from build123d import *

# Parameters (mm, degrees)
SKETCH1_W               = 160
SKETCH1_H               = 129
BOSS_EXTRUDE1_DEPTH     = 8
SKETCH1_3_R             = 4
CUT_EXTRUDE2_DEPTH      = 104.074002542
FILLET1_R               = 10
CUT_EXTRUDE4_DEPTH      = 1
CUT_EXTRUDE4_DEPTH_BACK = 3
CUT_EXTRUDE4_START      = 8
CUT_EXTRUDE9_DEPTH      = 104.074002542
CUT_EXTRUDE10_START     = 8
SKETCH1_17_R            = 2.5
SKETCH1_17_R_2          = 10
CUT_EXTRUDE10_DEPTH     = 5
BOSS_EXTRUDE4_START     = 10
BOSS_EXTRUDE4_DEPTH     = 10
FILLET2_R               = 10


with BuildPart() as part:
    # Sketch1 → Boss-Extrude1 (new body)
    with BuildSketch(Plane(origin=(0, 0, 0), x_dir=(1, 0, 0), z_dir=(0, 1, 0))):
        Rectangle(SKETCH1_W, SKETCH1_H)
    extrude(amount=BOSS_EXTRUDE1_DEPTH)

    # Sketch1<3> → Cut-Extrude2 (cut, through all)
    with BuildSketch(Plane(origin=(0, 0, 0), x_dir=(1, 0, 0), z_dir=(0, 1, 0))):
        with Locations(Location((-70, 54.5, 0), (0, 0, 270))):
            Circle(SKETCH1_3_R)
        with Locations(Location((-70, -54.5, 0), (0, 0, 270))):
            Circle(SKETCH1_3_R)
        with Locations(Location((70, -54.5, 0), (0, 0, 90))):
            Circle(SKETCH1_3_R)
        with Locations(Location((70, 54.5, 0), (0, 0, 90))):
            Circle(SKETCH1_3_R)
    extrude(amount=CUT_EXTRUDE2_DEPTH, mode=Mode.SUBTRACT)

    # Fillet1
    fillet1_edges = [part.edges().sort_by_distance(p)[0] for p in [
        (80, 4, 64.5),
        (-80, 4, 64.5),
        (-80, 4, -64.5),
        (80, 4, -64.5),
    ]]
    fillet(fillet1_edges, radius=FILLET1_R)

    # Sketch1<11> → Cut-Extrude4 (cut, two sides: drawn at the far end of the back side and taken through both)
    with BuildSketch(Plane(origin=(0, 0, 0), x_dir=(1, 0, 0), z_dir=(0, 1, 0)).offset(CUT_EXTRUDE4_START - CUT_EXTRUDE4_DEPTH_BACK)):
        with BuildLine():
            Line((53.875, -40.875), (-53.875, -40.875))
            ThreePointArc((-53.875, -40.875), (-58.824747468, -38.824747468), (-60.875, -33.875))
            Line((-60.875, -33.875), (-60.875, 33.875))
            ThreePointArc((-60.875, 33.875), (-58.824747468, 38.824747468), (-53.875, 40.875))
            Line((-53.875, 40.875), (53.875, 40.875))
            ThreePointArc((53.875, 40.875), (58.824747468, 38.824747468), (60.875, 33.875))
            Line((60.875, 33.875), (60.875, -33.875))
            ThreePointArc((60.875, -33.875), (58.824747468, -38.824747468), (53.875, -40.875))
        make_face()
    extrude(amount=CUT_EXTRUDE4_DEPTH + CUT_EXTRUDE4_DEPTH_BACK, mode=Mode.SUBTRACT)

    # Sketch1<13> → Cut-Extrude9 (cut, through all)
    with BuildSketch(Plane(origin=(0, 0, 0), x_dir=(1, 0, 0), z_dir=(0, 1, 0))):
        with BuildLine():
            Line((-70, -64.5), (70, -64.5))
            ThreePointArc((70, -64.5), (65.25658351, -63.303408431), (61.648353456, -60))
            Line((61.648353456, -60), (-61.648353456, -60))
            ThreePointArc((-61.648353456, -60), (-65.25658351, -63.303408431), (-70, -64.5))
        make_face()
        with BuildLine():
            ThreePointArc((61.648353456, 60), (65.25658351, 63.303408431), (70, 64.5))
            Line((70, 64.5), (-69.999999984, 64.5))
            ThreePointArc((-69.999999984, 64.5), (-65.256583502, 63.303408427), (-61.648353456, 60))
            Line((-61.648353456, 60), (61.648353456, 60))
        make_face()
    extrude(amount=CUT_EXTRUDE9_DEPTH, mode=Mode.SUBTRACT)

    # Sketch1<17> → Cut-Extrude10 (cut)
    with BuildSketch(Plane(origin=(0, 0, 0), x_dir=(1, 0, 0), z_dir=(0, 1, 0)).offset(CUT_EXTRUDE10_START)):
        with Locations(Location((0, 32.125, 0), (0, 0, 270))):
            Circle(SKETCH1_17_R)
        with Locations((-70, 54.5)):
            Circle(SKETCH1_17_R_2)
        with Locations((70, 54.5)):
            Circle(SKETCH1_17_R_2)
        with Locations((-70, -54.5)):
            Circle(SKETCH1_17_R_2)
        with Locations((70, -54.5)):
            Circle(SKETCH1_17_R_2)
        with Locations(Location((0, -33.625, 0), (0, 0, 270))):
            Circle(SKETCH1_17_R)
    extrude(amount=-CUT_EXTRUDE10_DEPTH, mode=Mode.SUBTRACT)

    # Sketch1<18> → Boss-Extrude4 (add)
    with BuildSketch(Plane(origin=(0, 0, 0), x_dir=(1, 0, 0), z_dir=(0, 1, 0)).offset(BOSS_EXTRUDE4_START)):
        with BuildLine():
            ThreePointArc((60.460607986, 57.5), (60.967568701, 58.791291743), (61.648353456, 60))
            Line((61.648353456, 60), (-61.648353456, 60))
            ThreePointArc((-61.648353456, 60), (-60.967568701, 58.791291743), (-60.460607986, 57.5))
            Line((-60.460607986, 57.5), (60.460607986, 57.5))
        make_face()
        with BuildLine():
            Line((-80, 54.500000177), (-80, -54.5))
            ThreePointArc((-80, -54.5), (-79.354143467, -50.964466094), (-77.5, -47.885621722))
            Line((-77.5, -47.885621722), (-77.5, 47.885621722))
            ThreePointArc((-77.5, 47.885621722), (-79.354143498, 50.964466177), (-80, 54.500000177))
        make_face()
        with BuildLine():
            ThreePointArc((77.5, -47.885621722), (79.354143467, -50.964466094), (80, -54.5))
            Line((80, -54.5), (80, 54.5))
            ThreePointArc((80, 54.5), (79.354143467, 50.964466094), (77.5, 47.885621722))
            Line((77.5, 47.885621722), (77.5, -47.885621722))
        make_face()
        with BuildLine():
            Line((-61.648353456, -60), (61.648353456, -60))
            ThreePointArc((61.648353456, -60), (60.967568701, -58.791291743), (60.460607986, -57.5))
            Line((60.460607986, -57.5), (-60.460607986, -57.5))
            ThreePointArc((-60.460607986, -57.5), (-60.967568701, -58.791291743), (-61.648353456, -60))
        make_face()
    extrude(amount=-BOSS_EXTRUDE4_DEPTH)

    # Fillet2
    # the kernel refuses this fillet: 10 mm, written as the material it adds along each edge
    with BuildSketch(Plane(origin=(61.648353456, 0, 60), x_dir=(0.6702455950029323, 0, 0.7421393685684416), z_dir=(0, 1, 0)), Plane(origin=(-61.648353456, 0, -60), x_dir=(-0.6702455950029282, 0, -0.7421393685684453), z_dir=(0, 1, 0))) as fillet2_piece_1:
        with BuildLine():
            CenterArc((4.547663341, -9.884436465), FILLET2_R, 98.719009802, 39.194967426)
            Line((-2.873730345, -3.181980515), (0, 0))
            ThreePointArc((0, 0), (1.51588778, -0.115563535), (3.03177556, 0))
        make_face()
    extrude(amount=3)
    with BuildSketch(Plane(origin=(-61.648353456, 0, 60), x_dir=(1, 0, 0), z_dir=(0, 1, 0))) as fillet2_piece_2:
        with BuildLine():
            CenterArc((4.287578116, -10), FILLET2_R, 90, 39.194967426)
            ThreePointArc((-2.032034214, -2.25), (-0.930252859, -1.20245595), (0, 0))
            Line((0, 0), (4.287578116, 0))
        make_face()
    extrude(amount=3)
    with BuildSketch(Plane(origin=(61.648353456, 0, -60), x_dir=(0.6702455950029361, 0, -0.7421393685684381), z_dir=(0, 1, 0))) as fillet2_piece_3:
        with BuildLine():
            CenterArc((4.547663341, 9.884436465), FILLET2_R, 222.086022772, 39.194967426)
            Line((-2.873730345, 3.181980515), (0, 0))
            ThreePointArc((0, 0), (1.51588778, 0.115563535), (3.03177556, 0))
        make_face()
    extrude(amount=3)


solid = part.part
Input: part model. Units: mm. Frame: model coordinates. A direction names the side the tool comes from. Coordinates: 2 decimals unless noted, no trailing zeros. Order: outer loops, then holes, each group sorted by start corner. A loop starts at its lowest first (then second) coordinate and runs counter-clockwise, first axis right, second up. Notation, with made-up numbers: M 62.5,38.25 L 75.5,38.25 A18 cw 75.5,62.25 Z; hole C 20.5,33 d11. An arc over 180 degrees is marked long. Answer as CSV lines item,"result".
1. Section B-B (y = 1.5). Return the cut outline in (x, z), then the cut area to 3 significant figures.
Reported:
outline,"M -80,-54.5 A10 ccw -63.68,-62.25 A10 cw -57.36,-60 L 57.36,-60 A10 cw 63.68,-62.25 A10 ccw 80,-54.5 L 80,54.5 A10 ccw 63.68,62.25 A10 cw 57.36,60 L -57.36,60 A10 cw -63.68,62.25 A10 ccw -80,54.5 Z; hole C -70,-54.5 d8; hole C -70,54.5 d8; hole C 70,-54.5 d8; hole C 70,54.5 d8"
area,"19,200 mm2"
2. First-contact query: P1, Ø6, axis at x = -24.5, z = -46, coming from the +Y side; P2, Ø1, axis at x = 1, y = 9, coming from the +Z side; P3, Ø5.5, axis at x = 0.5, z = -31.5, coming from the +Y side. Flat tips, straight axial feed; report the tip coordinate or a pass-through.
Reported:
P1,"y = 8"
P2,"z = 60"
P3,"y = 5"
3. Section A-A (x = 10). Return the cut outline in (y, z) (3 decimals), then the cut area to 3 significant figures.
Reported:
outline,"M 0,-60 L 10,-60 L 10,-57.5 L 8,-57.5 L 8,-40.875 L 5,-40.875 L 5,40.875 L 8,40.875 L 8,57.5 L 10,57.5 L 10,60 L 0,60 Z"
area,"725 mm2"
4. Material intervals for line 1 (X direction, y = 1, z = -54); line 2 (Z direction, x = 70, y = 2.5); line 3 (Z direction, x = 14.5, y = 7.75) (3 decimals), sorted ascending. Write a range as from..to.
Reported:
line 1,"-80..-73.97, -66.03..66.03, 73.97..80"
line 2,"-64.5..-58.5, -50.5..50.5, 58.5..64.5"
line 3,"-60..-40.875, 40.875..60"
5. Pull-direction query (Z, two-part tool) for faces 1 (the flat face through (0, 0, -2)), 2 (the flat face through (0, 3, -32)), 3 (the flat face through (1, 5, 60)); classes: released by +Z, released by -Z, zero draft, split by the parting line, or undercut.
Reported:
face 1,"zero draft"
face 2,"undercut"
face 3,"released by +Z"
6. Access query for faces 4 (the cylindrical face through (-73.549, 1.479, -52.654)), 5 (the flat face through (1, 5, -1)). Directions: +Z, -Z, +X, -X, +Y, -Y. A direction counts if a zero-diameter tool reaches every point of the face in a straight line with its end or side. Return the directions, or none.
Reported:
face 4,"+Y, -Y"
face 5,"+Y"
